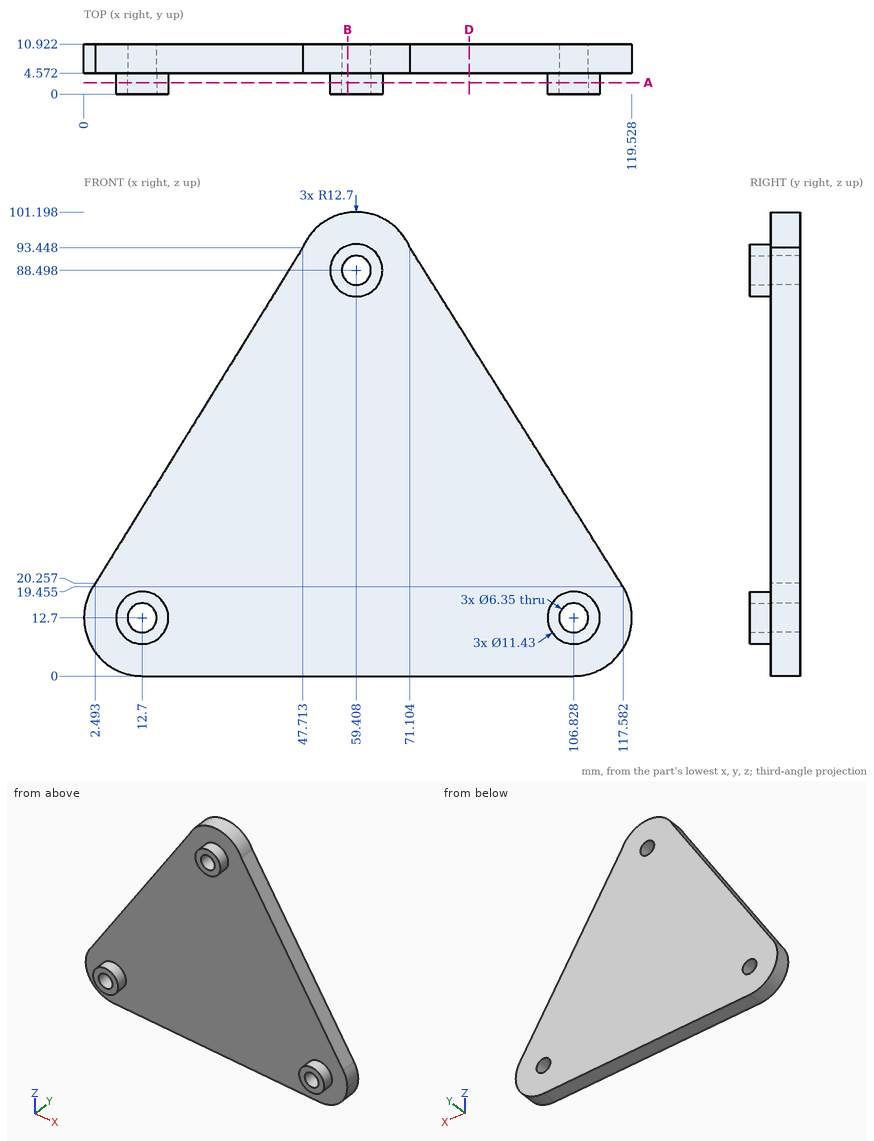
For this review, use the dimensioned drawing (mm, ordinates from the lowest corner) and the shaded views. Give positions to 0.01 mm unless a question says otherwise; leave off trailing zeros. Order: outer loops, then holes, each group sorted by start corner. A loop starts at its lowest first (then second) coordinate and runs counter-clockwise, first axis right, second up.
1) Take a section at D-D (x = 84). Give the boundary of the cut face in (y, z).
2) Wall thickness on line 1 (Z direction, x = 59, y = 10.25); line 2 (Z direction, x = 12.7, y = 3.3) (1 decimal); line 3 (Y direction, x = 7, z = 22): over which ranges is each line inside the solid? List them lowest first.
3) Insertion check: pin 1 (1 mm diameter, centred on y = 5.5, z = 63.5, fed in from +X); pin 2 (8.5 mm diameter, centred on x = 106.83, z = 12.7, fed in from +Y); pin 3 (5 mm diameter, centred on x = 47, z = 45, fed in from -Y); pin 4 (2 mm diameter, centred on y = 5, z = 66.5, fed in from +X). Each pin has a flat end and moves straight along its axis. Give the tip position at first contact, or say it passes through.
4) Take a section at B-B (x = 57.5). Give the boundary of the cut face in (y, z) (1 decimal).
5) Take a section at A-A (y = 2.5). State how many separate pieces and enclosed holes the cut face has, then the cut area to 3 significant figures.
Derived:
1. outline: (4.57, 0) - (10.92, 0) - (10.92, 72.92) - (4.57, 72.92) - close
2. line 1: z = 0 to 85.35, 91.65 to 101.19
2. line 2: z = 7 to 9.5, 15.9 to 18.4
2. line 3: y = 4.57 to 10.92
3. pin 1: stops at x = 90.23
3. pin 2: stops at y = 10.92
3. pin 3: stops at y = 4.57
3. pin 4: stops at x = 88.66
4. outline: (0, 83.1) - (4.6, 83.1) - (4.6, 0) - (10.9, 0) - (10.9, 86) - (0, 86) - close; (0, 91) - (10.9, 91) - (10.9, 101.1) - (4.6, 101.1) - (4.6, 93.9) - (0, 93.9) - close
5. separate pieces: 3
5. enclosed holes: 3
5. area: 213 mm2
